```python
from build123d import *

# Parameters (mm, degrees)
SKETCH1_W           = 35
SKETCH1_H           = 30
BOSS_EXTRUDE3_DEPTH = 5
SKETCH5_W           = 5
SKETCH5_H           = 30
BOSS_EXTRUDE4_DEPTH = 60
SKETCH6_R           = 2
SKETCH6_W           = 20.2
SKETCH6_H           = 41.2
CUT_EXTRUDE1_DEPTH  = 60
FILLET2_R           = 3
BOSS_EXTRUDE7_DEPTH = 5
FILLET3_R           = 6
SKETCH10_R          = 1.5
CUT_EXTRUDE2_DEPTH  = 5
FILLET4_R           = 6


with BuildPart() as part:
    # Sketch1 → Boss-Extrude3 (new body)
    with BuildSketch(Plane(origin=(0, 0, 0), x_dir=(1, 0, 0), z_dir=(0, 1, 0))):
        with Locations((17.5, 15)):
            Rectangle(SKETCH1_W, SKETCH1_H)
    extrude(amount=BOSS_EXTRUDE3_DEPTH)

    # Sketch5 → Boss-Extrude4 (add)
    with BuildSketch(Plane(origin=(0, 5, 0), x_dir=(1, 0, 0), z_dir=(0, 1, 0))):
        with Locations((2.5, 15)):
            Rectangle(SKETCH5_W, SKETCH5_H)
        with Locations((32.5, 15)):
            Rectangle(SKETCH5_W, SKETCH5_H)
    extrude(amount=BOSS_EXTRUDE4_DEPTH)

    # Sketch6 → Cut-Extrude1 (cut)
    with BuildSketch(Plane(origin=(35, 0, 0), x_dir=(0, 0, -1), z_dir=(1, 0, 0))):
        with Locations((10, 61)):
            Circle(SKETCH6_R)
        with Locations((20, 61)):
            Circle(SKETCH6_R)
        with Locations((10, 11.8)):
            Circle(SKETCH6_R)
        with Locations((20, 11.8)):
            Circle(SKETCH6_R)
        with Locations((15, 36.4)):
            Rectangle(SKETCH6_W, SKETCH6_H)
    extrude(amount=-CUT_EXTRUDE1_DEPTH, mode=Mode.SUBTRACT)

    # Fillet2
    fillet2_edges = [part.edges().sort_by_distance(p)[0] for p in [
        (5, 5, -15),
        (30, 5, -15),
    ]]
    fillet(fillet2_edges, radius=FILLET2_R)

    # Sketch8 → Boss-Extrude7 (add)
    with BuildSketch(Plane.ZY):
        with BuildLine():
            ThreePointArc((-30, 59), (-31.757359313, 63.242640687), (-36, 65))
            Line((-36, 65), (-36, 60.5))
            ThreePointArc((-36, 60.5), (-34.939339828, 60.060660172), (-34.5, 59))
            ThreePointArc((-34.5, 59), (-34.939339828, 57.939339828), (-36, 57.5))
            Line((-36, 57.5), (-36, 53))
            ThreePointArc((-36, 53), (-31.757359313, 54.757359313), (-30, 59))
        make_face()
        with BuildLine():
            Line((-36, 60.5), (-36, 65))
            ThreePointArc((-36, 65), (-42, 59), (-36, 53))
            Line((-36, 53), (-36, 57.5))
            ThreePointArc((-36, 57.5), (-37.5, 59), (-36, 60.5))
        make_face()
        with BuildLine():
            Line((-30, 59), (-30, 65))
            Line((-30, 65), (-36, 65))
            ThreePointArc((-36, 65), (-31.757359313, 63.242640687), (-30, 59))
        make_face()
        with BuildLine():
            Line((-30, 53), (-30, 59))
            ThreePointArc((-30, 59), (-31.757359313, 54.757359313), (-36, 53))
            Line((-36, 53), (-30, 53))
        make_face()
    extrude(amount=-BOSS_EXTRUDE7_DEPTH)

    # Fillet3
    fillet3_edges = [part.edges().sort_by_distance(p)[0] for p in [
        (2.5, 53, -30),
    ]]
    fillet(fillet3_edges, radius=FILLET3_R - 0.0001)  # a hair under: the kernel refuses the full size

    # Sketch10 → Cut-Extrude2 (cut)
    with BuildSketch(Plane(origin=(0, 5, 0), x_dir=(1, 0, 0), z_dir=(0, 1, 0))):
        with Locations(Location((17.5, 27.5, 0), (0, 0, 270))):
            Circle(SKETCH10_R)
        with Locations(Location((17.5, 2.5, 0), (0, 0, 270))):
            Circle(SKETCH10_R)
    extrude(amount=-CUT_EXTRUDE2_DEPTH, mode=Mode.SUBTRACT)

    # Fillet4
    fillet4_edges = [part.edges().sort_by_distance(p)[0] for p in [
        (2.5, 65, 0),
        (32.5, 65, -30),
        (32.5, 65, 0),
    ]]
    fillet(fillet4_edges, radius=FILLET4_R)


solid = part.part
```
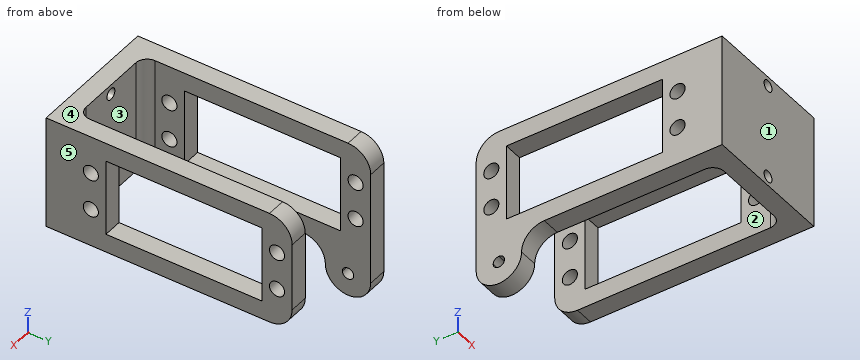
Build history of the part. All positions in model axes, mm. Face numbers are marked on the shaded views. A direction names the side the tool comes from. Round coordinates to 2 decimals unless told otherwise and drop trailing zeros. Write each loop counter-clockwise with the first axis right and the second up, starting at its lowest first coordinate (ties: lowest second). Pieces come first, ordered by that corner, then holes. Notation, with made-up numbers: (1, 22.5) - (59, 22.5) arc R18 cw to (59, 44.5) - close; hole circle Ø10 at (71, 52.25). An arc over 180 degrees is marked (long way). Write each question's results on one line, items separated by ' | '. Start each with the question number.
Item 1: Wall check: L1, parallel to Y at x = 1.2, z = -20; L2, parallel to X at y = 14, z = -9.5; L3, parallel to Z at x = 33, y = 33.5. Give the ranges that are in metal, low to high. Write a range as [from, to].
Item 2: Saw through at C-C (z = -20). State how many separate pieces and enclosed holes the cut face has, and give its area (3 significant figures).
Item 3: Saw through at B-B (x = 17.5). Write the cut outline in (y, z), and give its area (3 significant figures).
Item 4: Mould opens along X. For the marked faces 3, 4 and 5 say: pulls with the +X half, pulls with the -X half, needs draft (parallel to the pull), parting line crosses it, or undercut.
Item 5: Drop flat-ended pins along their axis: P1, Ø3, axis at y = 61, z = -20, coming from the +X side; P2, Ø1.5, axis at x = 31.5, y = 27, coming from the -Z side; P3, Ø12, axis at x = 13.5, z = -16.5, coming from the +Y side. Give the stop position or say it passes through.
Item 6: Saw through at D-D (y = 11.8). Write the cut outline in (x, z), and give its area (3 significant figures).
Item 7: Which spindle directions (+Z, -Z, +X, -X, +Y, -Y) get a long thin tool onto all of the face, cutting with end or side? Do the marked faces 1 and 2. Say none if no direction does.
Item 8: Saw through at A-A (y = 20.5). Write the cut outline in (x, z).
Results are:
1) L1: y = [0, 9.8], [13.8, 15.8], [57, 59], [63, 65] | L2: x = [0, 5], [30, 35] | L3: z = [-30, -25.1], [-4.9, 0]
2) separate pieces: 7 | enclosed holes: 0 | area: 287 mm²
3) outline: (0, -30) - (5, -30) - (5, -29) - (0, -29) - close; (0, -26) - (5, -26) - (5, -4) - (0, -4) - close; (0, -1) - (5, -1) - (5, 0) - (0, 0) - close | area: 120 mm²
4) face 3: undercut | face 4: needs draft | face 5: pulls with the +X half
5) P1: passes through | P2: stops at z = -30 | P3: stops at y = 5.04
6) outline: (0, -30) - (5, -30) - (5, -22) - (0, -22) - close; (0, -18) - (5, -18) - (5, -12) - (0, -12) - close; (0, -8) - (5, -8) - (5, 0) - (0, 0) - close; (30, -30) - (35, -30) - (35, -22) - (30, -22) - close; (30, -18) - (35, -18) - (35, -12) - (30, -12) - close; (30, -8) - (35, -8) - (35, 0) - (30, 0) - close | area: 220 mm²
7) face 1: +Z, -Z, +X, -X, -Y | face 2: +Z, -Z, +Y
8) outline: (0, -30) - (5, -30) - (5, -25.1) - (0, -25.1) - close; (0, -4.9) - (5, -4.9) - (5, 0) - (0, 0) - close; (30, -30) - (35, -30) - (35, -25.1) - (30, -25.1) - close; (30, -4.9) - (35, -4.9) - (35, 0) - (30, 0) - close
